```python
from build123d import *

# Parameters (mm, degrees)
F0_R     = 6.345
F0_W     = 4.3
F0_H     = 10.7
F1_DEPTH = 42
F2_DEPTH = 10


with BuildPart() as f1:
    # F0 (on Top) → F1 (new body)
    with BuildSketch(Plane.XY):
        Circle(F0_R)
        Rectangle(F0_W, F0_H, mode=Mode.SUBTRACT)
        Rectangle(F0_W, F0_H)
    extrude(amount=F1_DEPTH)

    # F0 (on Top) → F2 (join)
    with BuildSketch(Plane.XY):
        Rectangle(F0_W, F0_H)
    extrude(amount=-F2_DEPTH)


solid = f1.part
```
The model under review builds one solid part; all positions refer to its coordinate system, in mm. A direction names the side the tool comes from. Give positions to 0.01 mm unless a question says otherwise; leave off trailing zeros. Write each loop counter-clockwise with the first axis right and the second up, starting at its lowest first coordinate (ties: lowest second). Pieces come first, ordered by that corner, then holes. Notation, with made-up numbers: M 86,-30.5 L 133,-30.5 A37 ccw 133,8.5 Z; hole C 68.25,-37.75 d4. An arc over 180 degrees is marked long. Write item = value, one per line. Start each with the question number.
Q1. Clearance check with flat-ended pins moving along their axes: pin 1 (5 mm diameter, centred on y = -1, z = -3.5, fed in from +X); pin 2 (5 mm diameter, centred on x = -3, z = 29, fed in from +Y); pin 3 (1.5 mm diameter, centred on y = 4, z = 12.5, fed in from +X). State where each tip first meets the part, or that it passes through.
Q2. We need section C-C (z = 39). State the section outline as (x, y) points (3 decimals), plus the area to 3 significant figures.
Q3. Machinability: for faces 1 (the face through (0, 5.35, -5)), 2 (the face through (0, -5.35, -5)), 3 (the face through (2.15, 0, -5)), 4 (the face through (-2.15, 0, -5)), which of the approach directions +Z, -Z, +X, -X, +Y, -Y give a long, thin tool a straight path to every point of the face, cutting with its end or side? Answer none if there is none.
Q4. We need section A-A (y = 0). State the section outline as (x, z) points (3 decimals), plus the area to 3 significant figures.
Q5. We need section D-D (z = -4). State the section outline as (x, y) points.
Q6. For line 1 (X direction, y = 0, z = -3.5); line 2 (Z direction, x = -2.5, y = -4); line 3 (Y direction, x = -1, z = -6), list the stretches that pass through material, from the lowest coordinate up.
Q7. We need section B-B (x = 0). State the section outline as (y, z) points (3 decimals), plus the area to 3 significant figures.
Result set:
q1.pin_1 = 2.15
q1.pin_2 = 6.33
q1.pin_3 = 5.45
q2.outline = C 0,0 d12.69
q2.area = 126 mm2
q3.face_1 = -Z, +X, -X, +Y
q3.face_2 = -Z, +X, -X, -Y
q3.face_3 = -Z, +X, +Y, -Y
q3.face_4 = -Z, -X, +Y, -Y
q4.outline = M -6.345,0 L -2.15,0 L -2.15,-10 L 2.15,-10 L 2.15,0 L 6.345,0 L 6.345,42 L -6.345,42 Z
q4.area = 576 mm2
q5.outline = M -2.15,-5.35 L 2.15,-5.35 L 2.15,5.35 L -2.15,5.35 Z
q6.line_1 = -2.15 to 2.15
q6.line_2 = 0 to 42
q6.line_3 = -5.35 to 5.35
q7.outline = M -6.345,0 L -5.35,0 L -5.35,-10 L 5.35,-10 L 5.35,0 L 6.345,0 L 6.345,42 L -6.345,42 Z
q7.area = 640 mm2
